For this review, take the finished solid that the model builds, in its own axes (mm). Coordinates: 2 decimals unless noted, no trailing zeros. Write each loop counter-clockwise with the first axis right and the second up, starting at its lowest first coordinate (ties: lowest second). Pieces come first, ordered by that corner, then holes. Notation, with made-up numbers: M 2.25,27 L 61.25,27 A20 ccw 61.25,35 Z; hole C 1,84 d6. An arc over 180 degrees is marked long. Return JSON: item names as keys, results as strings.
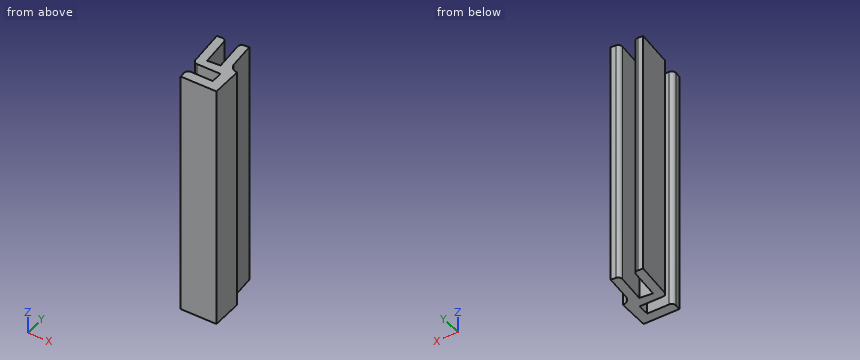
```python
from build123d import *

# Parameters (mm, degrees)
BOSS_EXTRUDE1_DEPTH = 38.1
CUT_EXTRUDE1_DEPTH  = 80.768105782
FILLET1_R           = 2.54
FILLET2_R           = 1.27


with BuildPart() as part:
    # Sketch1 → Boss-Extrude1 (new, symmetric)
    with BuildSketch(Plane.XY):
        Polygon((0, 0), (-11.03334096, 0), (-12.7, 19.05), (-3.211245501, 19.88015845), (-2.305286527, 9.525), (0, 9.525), align=None)
    extrude(amount=BOSS_EXTRUDE1_DEPTH, both=True)

    # Sketch2 → Cut-Extrude1 (cut, through all)
    with BuildSketch(Plane.XY.offset(38.1)):
        Polygon((-5.963233354, 19.63939071), (-5.077731008, 9.518052578), (-9.0625098, 9.169429607), (-9.948012147, 19.290767739), align=None)
        Polygon((-11.611116094, 6.604), (-3.175, 6.604), (-3.175, 3.048), (-11.300006406, 3.048), align=None)
    extrude(amount=-CUT_EXTRUDE1_DEPTH, mode=Mode.SUBTRACT)

    # Fillet1
    # the kernel refuses this fillet: 2.54 mm, written as the material it adds along each edge
    with BuildSketch(Plane(origin=(-2.305286527, 9.525, -38.1), x_dir=(1, 0, 0), z_dir=(0, 0, 1))) as fillet1_piece_1_section:
        with BuildLine():
            CenterArc((FILLET1_R * 0.916331174017, FILLET1_R), FILLET1_R, 185, 85)
            Line((-FILLET1_R * 0.0798635240743, FILLET1_R * 0.912844257252), (0, 0))
            Line((0, 0), (FILLET1_R * 0.916331174017, 0))
        make_face()
    fillet1_piece_1 = extrude(amount=76.2, mode=Mode.PRIVATE)
    fillet1_piece_1 = split(fillet1_piece_1, bisect_by=Plane(origin=(0, 10.045448834, 0), z_dir=(-1, 0, 0)), keep=Keep.TOP, mode=Mode.PRIVATE)
    add(fillet1_piece_1)

    # Fillet2
    fillet2_edges = [part.edges().sort_by_distance(p)[0] for p in [
        (-9.948012147, 19.290767739, 0),
        (-5.963233354, 19.63939071, 0),
        (-11.300006406, 3.048, 0),
        (-11.611116094, 6.604, 0),
    ]]
    fillet(fillet2_edges, radius=FILLET2_R)


solid = part.part
```
1. Clearance check with flat-ended pins moving along their axes: pin 1 Ø6 at (x, z) = (-9.5, -25.5) entering from +Y; pin 2 Ø6 at (y, z) = (16, -25.5) entering from -X; pin 3 Ø7.5 at (x, z) = (-6, 14.5) entering from +Y. State where each tip first meets the part, or that it passes through.
Checks:
{"pin 1": "y = 19.18", "pin 2": "x = -12.7", "pin 3": "y = 19.88"}
2. We need section B-B (y = 11). State the section outline as (x, z) points.
Checks:
{"outline": "M -12,-38.1 L -9.22,-38.1 L -9.22,38.1 L -12,38.1 Z; M -5.21,-38.1 L -2.28,-38.1 L -2.28,38.1 L -5.21,38.1 Z"}
3. We need section D-D (y = 5). State the section outline as (x, z) points (3 decimals).
Checks:
{"outline": "M -3.175,-38.1 L 0,-38.1 L 0,38.1 L -3.175,38.1 Z"}
4. We need section A-A (x = -7.75). State the section outline as (y, z) points, plus the area to 3 significant figures.
Checks:
{"outline": "M 0,-38.1 L 3.05,-38.1 L 3.05,38.1 L 0,38.1 Z; M 6.6,-38.1 L 9.28,-38.1 L 9.28,38.1 L 6.6,38.1 Z", "area": "436 mm2"}
5. Wall thickness on L1, parallel to Y at x = -4.75, z = -12.5; L2, parallel to Y at x = -7.25, z = -16; L3, parallel to X at y = 14, z = -2.5: over which ranges is each line inside the solid? List them lowest first. Write a range as from..to.
Checks:
{"L1": "0..3.05, 6.6..19.74", "L2": "0..3.05, 6.6..9.33", "L3": "-12.26..-9.49, -5.47..-2.7"}
